Autodesk Inventor part; units mm, degrees
ref_plane "YZ Plane" through (0, 0, 0) normal (1, 0, 0) x (0, 1, 0)
ref_plane "XZ Plane" through (0, 0, 0) normal (0, 1, 0) x (-1, 0, 0)
ref_plane "XY Plane" through (0, 0, 0) normal (0, 0, 1) x (1, 0, 0)
sketch "Sketch4" plane through (0, 0, 0) normal (0, 0, 1) x (1, 0, 0)
  line L0 (-2.1, 0) -> (8, 0)
  line L1 (0, 0) -> (-2.1, 0)
  line L2 (0, 2.5) -> (0, 1.725)
  line L3 (0.5, 1.225) -> (0.5, 1.225)
  line L4 (0.5, 1.225) -> (0.9, 1.25)
  arc A0 (0, 1.725) -> (0.5, 1.225) centre (0.5, 1.725) ccw
  line L5 (-2.1, 0) -> (-2.1, 1.25)
  line L6 (0, 2.5) -> (-1.1375, 2.5)
  arc A1 (-1.1375, 2.5) -> (-2.1, 1.25) centre (1.4883, -0.5175) ccw
  line L7 (0.9, 1.25) -> (8, 1.25)
  line L8 (8, 1.25) -> (8, 0)
  point P0 (0, 1.225)
  dimension "d71" = 0.5
  dimension "d72" = 8
  dimension "d74" = 0.4
  dimension "d75" = 2.45
  dimension "d78" = 2.5
  dimension "d82" = 4
  dimension "d83" = 2.1
  dimension "d84" = 5
  dimension "d104" = 7.1
  dimension "d105" = 2.5
revolve "Revolution7" add sketch "Sketch4" angle 360 about axis through (-2.1, 0, 0) along (1, 0, 0)
sketch "Sketch5" plane through (-2.1, 0, 0) normal (-1, 0, 0) x (0, 0, 1)
  circle A0 centre (0, 0) radius 1.2 construction
  circle A1 centre (0, 0) radius 0.84 construction
  line L0 (0, 0) -> (-0.7275, 0.42)
  line L1 (0, 0) -> (-0.7275, -0.42)
  line L2 (-1.8008, 0) -> (1.7887, 0)
  line L3 (-1.2, 0) -> (-0.7275, -0.42)
  line L4 (-1.2, 0) -> (-0.7275, 0.42)
  dimension "d88" = 2.4
  dimension "d89" = 1.68
  dimension "d90" = 30
  dimension "d91" = 30
extrude "Extrusion1" cut sketch "Sketch5" against normal blind 1.04
pattern_circular "Circular Pattern1" count 6 over 360 about axis through (-10, 0, 0) along (1, 0, 0) of "Extrusion1"
fillet "Fillet1" radius 0.24 12 edges at (-1.58, -1.0392, -0.6) (-1.58, -0.42, -0.7275) (-1.58, -0.84, 0) (-1.58, -1.0392, 0.6) (-1.58, -0.42, 0.7275) (-1.58, 0, 1.2) (-1.58, 0.84, 0) (-1.58, 1.0392, 0.6) (-1.58, 0.42, 0.7275) (-1.58, 0.42, -0.7275) (-1.58, 0, -1.2) (-1.58, 1.0392, -0.6)
thread "Thread7"
properties part number "Flachkopfschraube mit Innenrund ISO 14583 - M2,5 x 8 - 4.8" material "Stahl"
Could you check a few things on this model? Use its own coordinates, in mm. Round coordinates to 2 decimals unless told otherwise and drop trailing zeros. Loops run counter-clockwise (first coordinate to the right, second up) from the corner with the lowest first, then second, coordinate; pieces in that order, holes last. Notation, with made-up numbers: (-2, 86.25) - (21, 86.25) arc R11 ccw to (21, 92.25) - close; hole circle Ø10 at (2, 1). An arc over 180 degrees is marked (long way). Use CSV: the item, a comma, the result in double quotes.
Item 1: If we mould it in two halves opening along Z, with no side actions, what happens to faces 1 (the flat face through (-1.06, 0, 0)), 2 (the cylindrical face through (4.5, -0.27, -1.22)), 3 (the flat face through (0, 2, 1))? For each: pulls with the +Z half, pulls with the -Z half, needs draft (parallel to the pull), parting line crosses it, or undercut.
Here are the results:
face 1,"undercut"
face 2,"parting line crosses it"
face 3,"needs draft"
Item 2: Will these pins go through, and if not, where does the flat tip stop? pin 1 (0.6 mm diameter, centred on y = 0, z = 0.5, fed in from -X); pin 2 (1 mm diameter, centred on x = 2.5, y = 1.5, fed in from -Z).
Here are the results:
pin 1,"stops at x = -1.06"
pin 2,"stops at z = -0.75"
Item 3: If we section it at A-A on x = 4.75: List the corners of the cut face in (y, z) for me.
Here are the results:
outline,"circle Ø2.5 at (0, 0)"
Item 4: I need wall thicknesses on L1, parallel to Y at x = 4.25, z = 0.75; L2, parallel to Z at x = 6, y = -0.05; L3, parallel to Y at x = 2.5, z = 0.5. Which ranges of each line are inside material? Lowest first, please. Write a range as [from, to].
Here are the results:
L1,"y = [-1, 1]"
L2,"z = [-1.25, 1.25]"
L3,"y = [-1.15, 1.15]"
